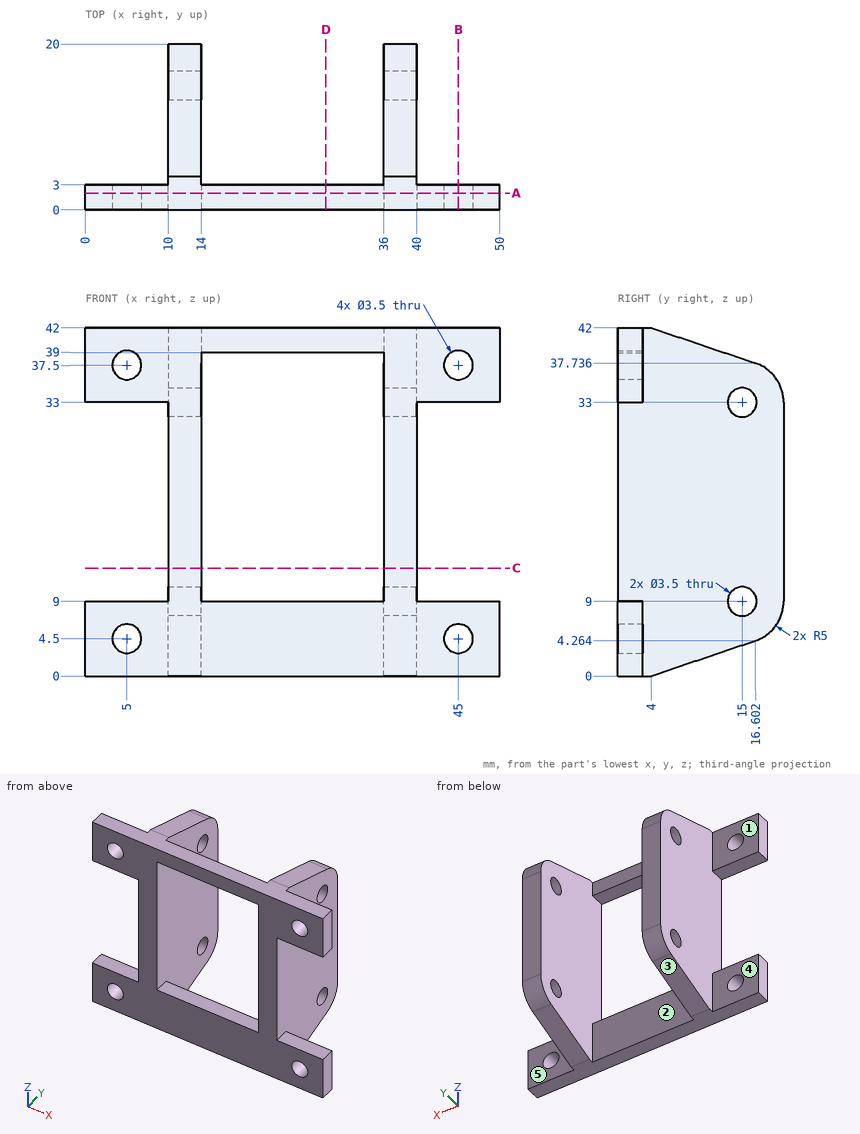
Part print with two shaded views. Sizes in mm from the minimum x, y, z corner. A direction names the side the tool comes from. Round coordinates to 2 decimals unless told otherwise and drop trailing zeros. Order: outer loops, then holes, each group sorted by start corner. A loop starts at its lowest first (then second) coordinate and runs counter-clockwise, first axis right, second up. Notation, with made-up numbers: M -20,44.5 L 31,44.5 A22 ccw 31,57.5 Z; hole C 75.25,84.5 d7. An arc over 180 degrees is marked long. Put each result on its own line as item: value. Start each with the question number.
1. Two-plate mould, pull along X, no slides. Class the marked faces 1 and 2: +X half, -X half, draft (parallel to the pull), parting line (faces both ways), or undercut.
2. Slice it at B-B on x = 45. List the corners of the cut face in (y, z).
3. Slice it at D-D on x = 29. List the corners of the cut face in (y, z), then the cut area to 3 significant figures.
4. Drop flat-ended pins along their axis: pin 1 (10 mm diameter, centred on y = 5.5, z = 22.5, fed in from -X); pin 2 (4 mm diameter, centred on x = 5, z = 37.5, fed in from +Y); pin 3 (3 mm diameter, centred on x = 13, y = 6.5, fed in from -Z). Give the stop position or say it passes through.
5. Drill centre lines: probe 1 along X at (y, z) = (0.8, 37.5); probe 2 along X at (y, z) = (2.25, 4.5); probe 3 along X at (y, z) = (11.5, 32.5). Where is each one in solid material? Low to high. Write a range as [from, to].
6. Slice it at A-A on y = 2. List the corners of the cut face in (x, z).
7. Slice it at C-C on z = 13. List the corners of the cut face in (x, y), then the cut area to 3 significant figures.
8. Tool access for the marked faces 3, 4 and 5: list every direction of +Z, -Z, +X, -X, +Y, -Y with a clear straight run to the whole face (end or side of a thin tool).
Findings:
1. face 1: draft
1. face 2: undercut
2. outline: M 0,0 L 3,0 L 3,2.75 L 0,2.75 Z; M 0,6.25 L 3,6.25 L 3,9 L 0,9 Z; M 0,33 L 3,33 L 3,35.75 L 0,35.75 Z; M 0,39.25 L 3,39.25 L 3,42 L 0,42 Z
3. outline: M 0,0 L 3,0 L 3,9 L 0,9 Z; M 0,39 L 3,39 L 3,42 L 0,42 Z
3. area: 36.0 mm2
4. pin 1: x = 10
4. pin 2: y = 3
4. pin 3: z = 0.34
5. probe 1: [0, 3.25], [6.75, 14], [36, 43.25], [46.75, 50]
5. probe 2: [0, 3.25], [6.75, 43.25], [46.75, 50]
5. probe 3: [10, 14], [36, 40]
6. outline: M 0,0 L 50,0 L 50,9 L 40,9 L 40,33 L 50,33 L 50,42 L 0,42 L 0,33 L 10,33 L 10,9 L 0,9 Z; hole C 5,4.5 d3.5; hole C 5,37.5 d3.5; hole M 14,9 L 36,9 L 36,39 L 14,39 Z; hole C 45,4.5 d3.5; hole C 45,37.5 d3.5
7. outline: M 10,0 L 14,0 L 14,20 L 10,20 Z; M 36,0 L 40,0 L 40,20 L 36,20 Z
7. area: 160 mm2
8. face 3: -Z, +X, -X, +Y
8. face 4: +Z, -Z, -X, +Y
8. face 5: +Z, -Z, +X, +Y
